```python
from build123d import *

# Parameters (mm, degrees)
SKETCH1_R                           = 17
BOSS_EXTRUDE1_DEPTH                 = 4.5
SKETCH2_R                           = 15
BOSS_EXTRUDE2_DEPTH                 = 1
SKETCH3_R                           = 15.5
BOSS_EXTRUDE3_DEPTH                 = 6
SKETCH7_R                           = 15
BOSS_EXTRUDE4_DEPTH                 = 8.5
SKETCH8_R                           = 12
BOSS_EXTRUDE5_DEPTH                 = 7.5
CUT_EXTRUDE1_REACH                  = 38.527
CUT_EXTRUDE1_END_RADIUS             = 15
SKETCH9_W                           = 3.5
SKETCH9_H                           = 3.5
CUT_EXTRUDE1_DIRECTION_2_REACH      = 38.527
CUT_EXTRUDE1_DIRECTION_2_END_RADIUS = 15
CHAMFER1_SIZE                       = 1
CHAMFER2_SIZE                       = 1
SKETCH10_R                          = 12.5
CUT_EXTRUDE2_DEPTH                  = 18
SKETCH11_R                          = 8
CUT_EXTRUDE3_DEPTH                  = 5
SKETCH12_R                          = 6.5
CUT_EXTRUDE4_DEPTH                  = 1
SKETCH13_R                          = 4.25
CUT_EXTRUDE5_DEPTH                  = 3.5
SKETCH17_W                          = 1
SKETCH17_H                          = 1.5
F_2_0_2_DIAMETER_HOLE1_D            = 2
F_2_0_2_DIAMETER_HOLE1_DEPTH        = 2.5
F_2_0_2_DIAMETER_HOLE1_TIP          = 0.600860619


with BuildPart() as part:
    # Sketch1 → Boss-Extrude1 (new body)
    with BuildSketch(Plane.XY):
        Circle(SKETCH1_R)
    extrude(amount=BOSS_EXTRUDE1_DEPTH)

    # Sketch2 → Boss-Extrude2 (add)
    with BuildSketch(Plane.XY.offset(4.5)):
        Circle(SKETCH2_R)
    extrude(amount=BOSS_EXTRUDE2_DEPTH)

    # Sketch3 → Boss-Extrude3 (add)
    with BuildSketch(Plane.XY.offset(5.5)):
        Circle(SKETCH3_R)
    extrude(amount=BOSS_EXTRUDE3_DEPTH)

    # Sketch7 → Boss-Extrude4 (add)
    with BuildSketch(Plane.XY.offset(11.5)):
        Circle(SKETCH7_R)
    extrude(amount=BOSS_EXTRUDE4_DEPTH)

    # Sketch8 → Boss-Extrude5 (add)
    with BuildSketch(Plane.XY.offset(20)):
        Circle(SKETCH8_R)
    extrude(amount=BOSS_EXTRUDE5_DEPTH)

    # Cut-Extrude1: up to this cylinder (the profile starts inside it)
    cut_extrude1_end = Plane(origin=(0, 0, 13.25), z_dir=(0, 0, -1)) * Cylinder(CUT_EXTRUDE1_END_RADIUS, 108.054, mode=Mode.PRIVATE)
    # Sketch9 → Cut-Extrude1 (cut, up to the surface)
    with BuildSketch(Plane(origin=(0, 0, 0), x_dir=(1, 0, 0), z_dir=(0, 1, 0)), mode=Mode.PRIVATE) as cut_extrude1_sk1:
        with Locations((0, -13.25)):
            Rectangle(SKETCH9_W, SKETCH9_H)
    cut_extrude1_tool1 = extrude(cut_extrude1_sk1.sketch, amount=-CUT_EXTRUDE1_REACH, mode=Mode.PRIVATE) & cut_extrude1_end
    add(cut_extrude1_tool1.solids().sort_by_distance((0, 0, 13.25))[0], mode=Mode.SUBTRACT)

    # Cut-Extrude1 direction 2: up to this cylinder (the profile starts inside it)
    cut_extrude1_direction_2_end = Plane(origin=(0, 0, 13.25), z_dir=(0, 0, -1)) * Cylinder(CUT_EXTRUDE1_DIRECTION_2_END_RADIUS, 108.054, mode=Mode.PRIVATE)
    # Sketch9 → Cut-Extrude1 direction 2 (cut, up to the surface)
    with BuildSketch(Plane(origin=(0, 0, 0), x_dir=(1, 0, 0), z_dir=(0, 1, 0)), mode=Mode.PRIVATE) as cut_extrude1_direction_2_sk1:
        with Locations((0, -13.25)):
            Rectangle(SKETCH9_W, SKETCH9_H)
    cut_extrude1_direction_2_tool1 = extrude(cut_extrude1_direction_2_sk1.sketch, amount=CUT_EXTRUDE1_DIRECTION_2_REACH, mode=Mode.PRIVATE) & cut_extrude1_direction_2_end
    add(cut_extrude1_direction_2_tool1.solids().sort_by_distance((0, 0, 13.25))[0], mode=Mode.SUBTRACT)

    # Chamfer1
    # the kernel refuses this chamfer: 1 mm, written as the material it takes off along each edge
    with BuildSketch(Plane(origin=(0, 0, 11.5), x_dir=(1, 0, 0), z_dir=(0, -1, 0))) as chamfer1_piece_1_section:
        Polygon((15.5, -CHAMFER1_SIZE), (15.5 - CHAMFER1_SIZE, 0), (15.5, 0), align=None)
    chamfer1_piece_1 = revolve(axis=Axis((0, 0, 11.5), (0, 0, 1)), mode=Mode.PRIVATE)
    chamfer1_piece_1 = chamfer1_piece_1 - Plane(origin=(0, 0, 10.7680681), x_dir=(1, 0, 0), z_dir=(0, 0, -1)) * Cylinder(15, 62, mode=Mode.PRIVATE)
    add(chamfer1_piece_1, mode=Mode.SUBTRACT)
    with BuildSketch(Plane(origin=(0, 0, 11.5), x_dir=(1, 0, 0), z_dir=(0, -1, 0))) as chamfer1_piece_2_section:
        Polygon((15.5, -CHAMFER1_SIZE), (15.5 - CHAMFER1_SIZE, 0), (15.5, 0), align=None)
    chamfer1_piece_2 = revolve(axis=Axis((0, 0, 11.5), (0, 0, 1)), mode=Mode.PRIVATE)
    chamfer1_piece_2 = split(chamfer1_piece_2, bisect_by=Plane(origin=(-1.75, 14.798779875, 11.333335543), z_dir=(1, 0, 0)), keep=Keep.TOP, mode=Mode.PRIVATE)
    chamfer1_piece_2 = split(chamfer1_piece_2, bisect_by=Plane(origin=(1.75, 14.798779875, 11.333335543), z_dir=(-1, 0, 0)), keep=Keep.TOP, mode=Mode.PRIVATE)
    add(chamfer1_piece_2, mode=Mode.SUBTRACT)

    # Chamfer2
    chamfer2_edges = [part.edges().sort_by_distance(p)[0] for p in [
        (-12, 0, 27.5),
    ]]
    chamfer(chamfer2_edges, length=CHAMFER2_SIZE)

    # Sketch10 → Cut-Extrude2 (cut)
    with BuildSketch(Plane(origin=(0, 0, 0), x_dir=(-1, 0, 0), z_dir=(0, 0, -1))):
        Circle(SKETCH10_R)
    extrude(amount=-CUT_EXTRUDE2_DEPTH, mode=Mode.SUBTRACT)

    # Sketch11 → Cut-Extrude3 (cut)
    with BuildSketch(Plane.XY.offset(27.5)):
        Circle(SKETCH11_R)
    extrude(amount=-CUT_EXTRUDE3_DEPTH, mode=Mode.SUBTRACT)

    # Sketch12 → Cut-Extrude4 (cut)
    with BuildSketch(Plane.XY.offset(22.5)):
        Circle(SKETCH12_R)
    extrude(amount=-CUT_EXTRUDE4_DEPTH, mode=Mode.SUBTRACT)

    # Sketch13 → Cut-Extrude5 (cut)
    with BuildSketch(Plane.XY.offset(21.5)):
        Circle(SKETCH13_R)
    extrude(amount=-CUT_EXTRUDE5_DEPTH, mode=Mode.SUBTRACT)

    # Sketch6 → Cut-Revolve4 (revolve, cut)
    with BuildSketch(Plane(origin=(0, 0, 0), x_dir=(0, 0, -1), z_dir=(1, 0, 0))):
        with BuildLine():
            Line((0, 14.5), (0, 15.6))
            Line((0, 15.6), (-1.560883383, 14.671907178))
            ThreePointArc((-1.560883383, 14.671907178), (-1.632511647, 14.598886259), (-1.658668305, 14.5))
            Line((-1.658668305, 14.5), (0, 14.5))
        make_face()
    revolve(axis=Axis((0, 14.5, 1.658668305), (0, 0, -1)), mode=Mode.SUBTRACT)

    # Sketch17 → Cut-Revolve5 (revolve, cut)
    with BuildSketch(Plane(origin=(0, 0, 0), x_dir=(0, 0, -1), z_dir=(1, 0, 0)), mode=Mode.PRIVATE) as cut_revolve5_sk:
        with Locations((-13.5, 14.25)):
            Rectangle(SKETCH17_W, SKETCH17_H)
    revolve(cut_revolve5_sk.sketch.rotate(Axis((0, 0, 0), (0, 0, 1)), 6.699765178), axis=Axis((0, 0, 0), (0, 0, 1)), mode=Mode.SUBTRACT)

    # Ø2.0 (2) Diameter Hole1
    with Locations(Plane(origin=(0, 0, 18), x_dir=(-1, 0, 0), z_dir=(0, 0, -1))):
        with Locations((0, 8.5), (7.361215932, -4.25), (-7.361215932, -4.25)):
            Hole(F_2_0_2_DIAMETER_HOLE1_D / 2, depth=F_2_0_2_DIAMETER_HOLE1_DEPTH)
            with Locations((0, 0, -(F_2_0_2_DIAMETER_HOLE1_DEPTH + F_2_0_2_DIAMETER_HOLE1_TIP / 2))):  # 118° drill point
                Cone(0, F_2_0_2_DIAMETER_HOLE1_D / 2, F_2_0_2_DIAMETER_HOLE1_TIP, mode=Mode.SUBTRACT)


solid = part.part
```
The listing builds one solid part. Answer for the finished solid, in the listing's coordinates (mm). A direction names the side the tool comes from. Give positions to 0.01 mm unless a question says otherwise; leave off trailing zeros. Order: outer loops, then holes, each group sorted by start corner. A loop starts at its lowest first (then second) coordinate and runs counter-clockwise, first axis right, second up. Notation, with made-up numbers: M 13.25,73.5 L 54.25,73.5 A19 cw 54.25,86.5 Z; hole C -31.75,-27.5 d8. An arc over 180 degrees is marked long. Put each result on its own line as item: value. Start each with the question number.
Item 1: Which of the six approach directions +Z, -Z, +X, -X, +Y, -Y give full straight-line access (tool end or side, diameter ignored) to faces 4 (the face through (6, -14, 4.5)), 5 (the face through (-15, 0, 12)), 6 (the face through (8.3, -3.9, 19.3)), 7 (the face through (-14.985, 0.66, 16.958)), 8 (the face through (0, 13, 11.5))?
Item 2: For a pull along X with two mould halves and no side action, classify faces 1 (the face through (-0.13, 9.49, 19.27)), 2 (the face through (-2.018, 15.368, 7.965)), 3 (the face through (13.497, -0.272, 13.493)) as +X half, -X half, draft (parallel to the pull), parting line (faces both ways), or undercut.
Item 3: Find the intervals of material crossed by line 1 along Y through (x, z) = (0, 19.55); line 2 along Y through (x, z) = (0, 25.55); line 3 along Y through (x, z) = (0, 22), in increasing order.
Item 4: The part is cut by section B-B, the plane z = 13.5. Determine the outline of the cut face in (x, y).
Item 5: The part is cut by section A-A, the plane z = 19.5. Determine the outline of the cut face in (x, y).
Item 6: The part is cut by section C-C, the plane z = 25. Determine the outline of the cut face in (x, y).
Item 7: Flat-ended cylindrical pins translate along their axes: P1, Ø10.5, axis at x = 8.5, y = -6.5, coming from the -Z side; P2, Ø5, axis at x = 0, y = 0, coming from the +Z side; P3, Ø15, axis at x = 0, y = 0, coming from the +Z side; P4, Ø4, axis at x = -5.5, y = -3.5, coming from the -Z side. Find the tip coordinate at first contact, or state that the pin passes through.
Item 8: The part is cut by section D-D, the plane z = 8. Determine the outline of the cut face in (x, y).
Answer key:
1. face 4: none
1. face 5: +Z, -X
1. face 6: -Z
1. face 7: +Z
1. face 8: +Y, -Y
2. face 1: undercut
2. face 2: parting line
2. face 3: +X half
3. line 1: y = -15 to -4.25, 4.25 to 7.5, 9.5 to 15
3. line 2: y = -12 to -8, 8 to 12
3. line 3: y = -12 to -6.5, 6.5 to 12
4. outline: M -1.75,-13.39 L -1.75,-12.38 A12.5 cw -1.75,12.38 L -1.75,13.39 A13.5 ccw Z; M 1.75,-13.39 A13.5 ccw 1.75,13.39 L 1.75,12.38 A12.5 cw 1.75,-12.38 Z
5. outline: C 0,0 d30; hole C -7.36,-4.25 d2; hole C 0,0 d8.5; hole C 0,8.5 d2; hole C 7.36,-4.25 d2
6. outline: C 0,0 d24; hole C 0,0 d16
7. P1: stops at z = 0
7. P2: passes through
7. P3: stops at z = 22.5
7. P4: stops at z = 18
8. outline: C 0,0 d31; hole C 0,0 d25
